```python
from build123d import *

# Parameters (mm, degrees)
SKETCH1_R                = 7.5
SKETCH1_R_2              = 5
BOSS_EXTRUDE1_DEPTH      = 18
BOSS_EXTRUDE1_DEPTH_BACK = 18
SKETCH3_R                = 10
SKETCH2_R                = 7.5
SKETCH4_R                = 10
SKETCH4_R_2              = 8
BOSS_EXTRUDE3_DEPTH      = 28
SKETCH5_R                = 11.643608711
SKETCH5_R_2              = 8
BOSS_EXTRUDE4_DEPTH      = 1


with BuildPart() as part:
    # Sketch1 → Boss-Extrude1 (new body, two sides)
    with BuildSketch(Plane.XY) as boss_extrude1_sk:
        Circle(SKETCH1_R)
        Circle(SKETCH1_R_2, mode=Mode.SUBTRACT)
    extrude(amount=BOSS_EXTRUDE1_DEPTH)
    extrude(boss_extrude1_sk.sketch, amount=-BOSS_EXTRUDE1_DEPTH_BACK)

    # Sketch3 → Loft1 section 0
    with BuildSketch(Plane(origin=(0, 10, 0), x_dir=(1, 0, 0), z_dir=(0, 1, 0))):
        Circle(SKETCH3_R)
    # Sketch2 → Loft1 section 1
    with BuildSketch(Plane(origin=(0, 0, 0), x_dir=(1, 0, 0), z_dir=(0, 1, 0))):
        Circle(SKETCH2_R)
    loft()

    # Sketch4 → Boss-Extrude3 (add)
    with BuildSketch(Plane(origin=(0, 10, 0), x_dir=(1, 0, 0), z_dir=(0, 1, 0))):
        Circle(SKETCH4_R)
        Circle(SKETCH4_R_2, mode=Mode.SUBTRACT)
    extrude(amount=BOSS_EXTRUDE3_DEPTH)

    # Sketch5 → Boss-Extrude4 (add)
    with BuildSketch(Plane(origin=(0, 38, 0), x_dir=(1, 0, 0), z_dir=(0, 1, 0))):
        Circle(SKETCH5_R)
        Circle(SKETCH5_R_2, mode=Mode.SUBTRACT)
    extrude(amount=BOSS_EXTRUDE4_DEPTH)


solid = part.part
```
Geometry check sheet. Reference: the model listing, model coordinates, mm. A direction names the side the tool comes from. Give positions to 0.01 mm unless a question says otherwise; leave off trailing zeros. Order: outer loops, then holes, each group sorted by start corner. A loop starts at its lowest first (then second) coordinate and runs counter-clockwise, first axis right, second up. Notation, with made-up numbers: (38, 3) - (74, 3) arc R19 cw to (74, 37) - close; hole circle Ø10 at (18.25, -12.5). An arc over 180 degrees is marked (long way). Answer in a Markdown table with one row per item. Add a question column.
Q1. Mould release check, pull along Y, two halves, no side actions. Record for faces 1 (the cylindrical face through (-2.524, 38.493, 11.367)), 2 (the flat face through (-3, 39, 8)), 3 (the flat face through (5, 38, -9)), 4 (the cylindrical face through (-2.17, 23.8, 9.76)): pulls with the +Y half, pulls with the -Y half, needs draft (parallel to the pull), parting line crosses it, or undercut.
Q2. Tool access check on faces 5 (the flat face through (2, -5, 18)), 6 (the cylindrical face through (-1.63, -7.32, 0.25)), 7 (the flat face through (0, 0, 0)), 8 (the flat face through (0, 10, 0)), 9 (the flat face through (2, -5, -18)). Record the directions out of +Z, -Z, +X, -X, +Y, -Y that give a thin tool (end or side, any length) a straight path to the whole face; none if there is none.
Q3. Cross-section at A-A, the plane y = 29.5. Enter the section's corners in (x, z), then the cut area to 3 significant figures.
Q4. Material ranges on probe 1 along Y at (x, z) = (0, 10.75); probe 2 along X at (y, z) = (19, 0); probe 3 along Y at (x, z) = (0, 5.75), recorded low to high. Write a range as from..to.
Q5. Gauge pin test, flat ends, axial feed: pin 1 (12 mm diameter, centred on y = 21, z = 11.5, fed in from +X); pin 2 (10 mm diameter, centred on y = 28, z = 4.5, fed in from +X); pin 3 (1.5 mm diameter, centred on x = -7, y = 6, fed in from +Z); pin 4 (5 mm diameter, centred on x = -2.5, z = 2.5, fed in from -Y). Record the tip position at first contact, or that the pin passes through.
Q6. Cross-section at D-D, the plane y = 6.5. Enter the section's corners in (x, z) (3 decimals).
Q7. Cross-section at C-C, the plane x = 0. Enter the section's corners in (y, z) (3 decimals).
Q8. Cross-section at B-B, the plane z = 16. Enter the section's corners in (x, y), then the cut area to 3 significant figures.
Check values:
| question | item | result |
|---|---|---|
| 1 | face 1 | needs draft |
| 1 | face 2 | pulls with the +Y half |
| 1 | face 3 | undercut |
| 1 | face 4 | undercut |
| 2 | face 5 | +Z, +X, -X, +Y, -Y |
| 2 | face 6 | none |
| 2 | face 7 | +Z, -Z |
| 2 | face 8 | +Y |
| 2 | face 9 | -Z, +X, -X, +Y, -Y |
| 3 | outline | circle Ø20 at (0, 0); hole circle Ø16 at (0, 0) |
| 3 | area | 113 mm^2 |
| 4 | probe 1 | y = -7.5..-5, 5..7.5, 38..39 |
| 4 | probe 2 | x = -10..-8, 8..10 |
| 4 | probe 3 | y = -7.5..-5, 0..10 |
| 5 | pin 1 | stops at x = 8.35 |
| 5 | pin 2 | stops at x = 10 |
| 5 | pin 3 | stops at z = 6.52 |
| 5 | pin 4 | stops at y = -7.5 |
| 6 | outline | (-3.742, -18) - (3.742, -18) - (3.742, -8.323) arc R9.125 ccw to (3.742, 8.323) - (3.742, 18) - (-3.742, 18) - (-3.742, 8.323) arc R9.125 ccw to (-3.742, -8.323) - close |
| 7 | outline | (-7.5, -18) - (-5, -18) - (-5, 18) - (-7.5, 18) - close; (0, -7.5) - (5, -8.75) - (5, -18) - (7.5, -18) - (7.5, -9.375) - (10, -10) - (38, -10) - (38, -11.644) - (39, -11.644) - (39, -8) - (10, -8) - (10, 8) - (39, 8) - (39, 11.644) - (38, 11.644) - (38, 10) - (10, 10) - (7.5, 9.375) - (7.5, 18) - (5, 18) - (5, 8.75) - (0, 7.5) - close |
| 8 | outline | circle Ø15 at (0, 0); hole circle Ø10 at (0, 0) |
| 8 | area | 98.2 mm^2 |
